Read the model definition and answer for the solid it produces. Units are mm, in the model's axes. A direction names the side the tool comes from. Give positions to 0.01 mm unless a question says otherwise; leave off trailing zeros. Write each loop counter-clockwise with the first axis right and the second up, starting at its lowest first coordinate (ties: lowest second). Pieces come first, ordered by that corner, then holes. Notation, with made-up numbers: (-14, 63.5) - (31, 63.5) arc R12 cw to (31, 69.5) - close; hole circle Ø1 at (56, 82.5). An arc over 180 degrees is marked (long way). Answer as a JSON object with one key per item and string values. Group by question number.
```python
from build123d import *

# Parameters (mm, degrees)
SKETCH1_W                = 4
SKETCH1_H                = 30
REVOLVE1_ANGLE           = 180
BOSS_EXTRUDE3_DEPTH      = 5
BOSS_EXTRUDE3_DEPTH_BACK = 5
SKETCH6_W                = 8.13
SKETCH6_H                = 5
M3_CLEARANCE_HOLE1_D     = 3.4
M3_CLEARANCE_HOLE1_DEPTH = 8.87
M3_CLEARANCE_HOLE1_TIP   = 1.021463052
SKETCH11_W               = 62.08504313
SKETCH11_H               = 41.873291452
CUT_EXTRUDE1_DEPTH       = 1


with BuildPart() as part:
    # Sketch1 → Revolve1 (revolve)
    with BuildSketch(Plane(origin=(0, 0, 0), x_dir=(1, 0, 0), z_dir=(0, 1, 0))):
        with Locations((-19.87, 0)):
            Rectangle(SKETCH1_W, SKETCH1_H)
    revolve(axis=Axis((0, 0, -19.621046531), (0, 0, 1)), revolution_arc=REVOLVE1_ANGLE)

    # Sketch6 → Boss-Extrude3 (add, two sides: drawn at the far end of the back side and taken through both)
    with BuildSketch(Plane.XY.offset(-BOSS_EXTRUDE3_DEPTH_BACK)):
        with Locations((-23.935, -2.5)):
            Rectangle(SKETCH6_W, SKETCH6_H)
        with Locations((23.935, -2.5)):
            Rectangle(SKETCH6_W, SKETCH6_H)
    extrude(amount=BOSS_EXTRUDE3_DEPTH + BOSS_EXTRUDE3_DEPTH_BACK)

    # M3 Clearance Hole1
    with Locations(Plane(origin=(0, 0, 0), x_dir=(1, 0, 0), z_dir=(0, 1, 0))):
        with Locations((-23.970037453, 0), (23.778277154, 0)):
            Hole(M3_CLEARANCE_HOLE1_D / 2, depth=M3_CLEARANCE_HOLE1_DEPTH)
            with Locations((0, 0, -(M3_CLEARANCE_HOLE1_DEPTH + M3_CLEARANCE_HOLE1_TIP / 2))):  # 118° drill point
                Cone(0, M3_CLEARANCE_HOLE1_D / 2, M3_CLEARANCE_HOLE1_TIP, mode=Mode.SUBTRACT)

    # Sketch11 → Cut-Extrude1 (cut)
    with BuildSketch(Plane(origin=(0, 0, 0), x_dir=(1, 0, 0), z_dir=(0, 1, 0))):
        Rectangle(SKETCH11_W, SKETCH11_H)
    extrude(amount=-CUT_EXTRUDE1_DEPTH, mode=Mode.SUBTRACT)


solid = part.part
```
1) For a pull along Z with two mould halves and no side action, classify faces 4 (the cylindrical face through (25.477, -3.028, -0.075)), 5 (the flat face through (-25, -3, 5)), 6 (the flat face through (-28, -3, 0)) as released by +Z, released by -Z, zero draft, split by the parting line, or undercut.
2) Find the intervals of material crossed by line 1 (X direction, y = -7.75, z = -10); line 2 (X direction, y = -6.5, z = -7.5); line 3 (Y direction, x = 25, z = 4), in increasing order. Write a range as [from, to].
3) Find section A-A, the plane z = 0. Write down the section's boundary in (x, y).
4) Which of the six approach directions +Z, -Z, +X, -X, +Y, -Y give full straight-line access (tool end or side, diameter ignored) to faces 1 (the flat face through (-25.4, -5, -1.2)), 2 (the flat face through (25.3, -5, -1.2)), 3 (the flat face through (21.7, -1, -0.2))?
5) Find section B-B, the plane y = -8.25. Write down the section's boundary in (x, z), and give its area (3 significant figures).
6) Flat-ended cylindrical pins translate along their axes: pin 1 Ø3.5 at (x, z) = (25, 0.5) entering from -Y; pin 2 Ø5 at (y, z) = (-13.5, 5) entering from +X; pin 3 Ø1.2 at (x, y) = (-25.5, -2.5) entering from -Z. Find the tip coordinate at first contact, or state that the pin passes through.
7) Find section C-C, the plane z = 4. Write down the section's boundary in (x, y).
8) Find section D-D, the plane x = 0. Write down the section's boundary in (y, z).
Values follow:
{
 "1": {"face 4": "undercut", "face 5": "released by +Z", "face 6": "zero draft"},
 "2": {"line 1": "x = [-20.45, -16.1], [16.1, 20.45]", "line 2": "x = [-20.88, -16.65], [16.65, 20.88]", "line 3": "y = [-5, -1]"},
 "3": {"outline": "(-28, -5) - (-25.67, -5) - (-25.67, -1) - (-28, -1) - close; (-22.27, -5) - (-21.29, -5) arc R21.87 ccw to (21.29, -5) - (22.08, -5) - (22.08, -1) - (17.84, -1) arc R17.87 cw to (-17.84, -1) - (-22.27, -1) - close; (25.48, -5) - (28, -5) - (28, -1) - (25.48, -1) - close"},
 "4": {"face 1": "+Z, -Z, -X, -Y", "face 2": "+Z, -Z, +X, -Y", "face 3": "+Z, -Z, +X, -X, +Y"},
 "5": {"outline": "(-20.25, -15) - (-15.85, -15) - (-15.85, 15) - (-20.25, 15) - close; (15.85, -15) - (20.25, -15) - (20.25, 15) - (15.85, 15) - close", "area": "264 mm2"},
 "6": {"pin 1": "stops at y = -5", "pin 2": "stops at x = 18.9", "pin 3": "stops at z = -5"},
 "7": {"outline": "(-28, -5) - (-21.29, -5) arc R21.87 ccw to (21.29, -5) - (28, -5) - (28, -1) - (17.84, -1) arc R17.87 cw to (-17.84, -1) - (-28, -1) - close"},
 "8": {"outline": "(-21.87, -15) - (-17.87, -15) - (-17.87, 15) - (-21.87, 15) - close"}
}
